The listing builds one solid part. Answer for the finished solid, in the listing's coordinates (mm). A direction names the side the tool comes from. Round coordinates to 2 decimals unless told otherwise and drop trailing zeros. Order: outer loops, then holes, each group sorted by start corner. A loop starts at its lowest first (then second) coordinate and runs counter-clockwise, first axis right, second up. Notation, with made-up numbers: (-26.75, 6.25) -> (28.25, 6.25) arc R19 ccw to (28.25, 12.25) -> close; hole circle Ø10 at (0, 2.5). An arc over 180 degrees is marked (long way). Return JSON: item names as keys, results as strings. Group by question number.
(1) Which of the six approach directions +Z, -Z, +X, -X, +Y, -Y give full straight-line access (tool end or side, diameter ignored) to faces 5 (the face through (-27.5, 15, 0)), 6 (the face through (0, 2.5, 0))?
(2) The part is cut by section A-A (x = -10.5). Determine the outline of the cut face in (y, z).
(3) Determine the mould class of faces 1 (the face through (25, 15, 0)), 2 (the face through (-18.422, 28.768, -0.338)), 3 (the face through (-25, 15, 0)), 4 (the face through (0, 30, 0)) for opening direction Y: +Y half, -Y half, draft (parallel to the pull), parting line (faces both ways), or undercut.
(4) The part is cut by section B-B (y = 11.25). Determine the outline of the cut face in (x, z).
(5) Consider line 1 (X direction, y = 28.15, z = 0); line 2 (Y direction, x = -9.5, z = 0.75); line 3 (X direction, y = 11, z = 0.5). Determine where each line is inside the solid, lowest interval first. Write a range as [from, to].
(6) The part is cut by section C-C (z = -8.25). Determine the outline of the cut face in (x, y).
(7) The part is cut by section D-D (x = -21). Determine the outline of the cut face in (y, z), plus the area to 3 significant figures.
from build123d import *

# Parameters (mm, degrees)
SKETCH_1_W          = 55
SKETCH_1_H          = 20
EXTRUDE_1_DEPTH     = 30
CUT_EXTRUDE_1_REACH = 47.346
SKETCH_2_W          = 50
SKETCH_2_H          = 25
CUT_EXTRUDE_2_REACH = 43.908
SKETCH_3_R          = 2.6


with BuildPart() as part:
    # 草图1 → 凸台-拉伸1 (new body)
    with BuildSketch(Plane(origin=(0, 0, 0), x_dir=(1, 0, 0), z_dir=(0, 1, 0))):
        Rectangle(SKETCH_1_W, SKETCH_1_H)
    extrude(amount=EXTRUDE_1_DEPTH)

    # 草图2 → 切除-拉伸1 (cut, up to next)
    with BuildSketch(Plane.XY.offset(10), mode=Mode.PRIVATE) as cut_extrude_1_sk1:
        with Locations((0, 15)):
            Rectangle(SKETCH_2_W, SKETCH_2_H)
    cut_extrude_1_tool1 = extrude(cut_extrude_1_sk1.sketch, amount=-CUT_EXTRUDE_1_REACH, mode=Mode.PRIVATE) & part.part
    add(cut_extrude_1_tool1.solids().sort_by_distance((0, 15, 10))[0], mode=Mode.SUBTRACT)

    # 切除-拉伸2: up to this face of the body (flat: up to its plane)
    cut_extrude_2_end = Plane(part.part.faces().sort_by_distance((0, 0, 0))[0])
    # 草图3 → 切除-拉伸2 (cut, up to the picked face)
    with BuildSketch(Plane(origin=(0, 30, 0), x_dir=(1, 0, 0), z_dir=(0, 1, 0)), mode=Mode.PRIVATE) as cut_extrude_2_sk1:
        with Locations(Location((-21, 0, 0), (0, 0, 270))):
            Circle(SKETCH_3_R)
    cut_extrude_2_tool1 = split(extrude(cut_extrude_2_sk1.sketch, amount=-CUT_EXTRUDE_2_REACH, mode=Mode.PRIVATE), bisect_by=cut_extrude_2_end, keep=Keep.BOTH, mode=Mode.PRIVATE)
    # 草图3 → 切除-拉伸2 (cut, up to the picked face)
    with BuildSketch(Plane(origin=(0, 30, 0), x_dir=(1, 0, 0), z_dir=(0, 1, 0)), mode=Mode.PRIVATE) as cut_extrude_2_sk2:
        with Locations(Location((21, 0, 0), (0, 0, 270))):
            Circle(SKETCH_3_R)
    cut_extrude_2_tool2 = split(extrude(cut_extrude_2_sk2.sketch, amount=-CUT_EXTRUDE_2_REACH, mode=Mode.PRIVATE), bisect_by=cut_extrude_2_end, keep=Keep.BOTH, mode=Mode.PRIVATE)
    add(cut_extrude_2_tool1.solids().sort_by(Axis((-21, 30, 0), (0, -1, 0)))[0], mode=Mode.SUBTRACT)
    add(cut_extrude_2_tool2.solids().sort_by(Axis((21, 30, 0), (0, -1, 0)))[0], mode=Mode.SUBTRACT)


solid = part.part
Answer below:
{
 "1": {"face 5": "+Z, -Z, -X, +Y, -Y", "face 6": "+Z, -Z"},
 "2": {"outline": "(0, -10) -> (2.5, -10) -> (2.5, 10) -> (0, 10) -> close; (27.5, -10) -> (30, -10) -> (30, 10) -> (27.5, 10) -> close"},
 "3": {"face 1": "undercut", "face 2": "draft", "face 3": "undercut", "face 4": "+Y half"},
 "4": {"outline": "(-27.5, -10) -> (-25, -10) -> (-25, 10) -> (-27.5, 10) -> close; (25, -10) -> (27.5, -10) -> (27.5, 10) -> (25, 10) -> close"},
 "5": {"line 1": "x = [-27.5, -23.6], [-18.4, 18.4], [23.6, 27.5]", "line 2": "y = [0, 2.5], [27.5, 30]", "line 3": "x = [-27.5, -25], [25, 27.5]"},
 "6": {"outline": "(-27.5, 0) -> (27.5, 0) -> (27.5, 30) -> (-27.5, 30) -> close; hole (-25, 2.5) -> (25, 2.5) -> (25, 27.5) -> (-25, 27.5) -> close"},
 "7": {"outline": "(0, -10) -> (2.5, -10) -> (2.5, -2.6) -> (0, -2.6) -> close; (0, 2.6) -> (2.5, 2.6) -> (2.5, 10) -> (0, 10) -> close; (27.5, -10) -> (30, -10) -> (30, -2.6) -> (27.5, -2.6) -> close; (27.5, 2.6) -> (30, 2.6) -> (30, 10) -> (27.5, 10) -> close", "area": "74.0 mm²"}
}
